```python
from build123d import *

# Parameters (mm, degrees)
EXTRUDE_1_DEPTH          = 16.25
EXTRUDE_1_DEPTH_BACK     = 16.25
SKETCH_2_R               = 1.5
CUT_EXTRUDE_1_DEPTH      = 39.484574832
CUT_EXTRUDE_1_DEPTH_BACK = 39.484574832
SKETCH_3_R               = 1
FILLET_1_R               = 2
CHAMFER_1_SIZE           = 1
SKETCH_4_W               = 8.5
SKETCH_4_H               = 4
CUT_EXTRUDE_2_DEPTH      = 39.484574832


with BuildPart() as part:
    # Sketch 2 → Extrude 1 (new, two sides: drawn at the far end of the back side and taken through both)
    with BuildSketch(Plane(origin=(0, 0, 0), x_dir=(1, 0, 0), z_dir=(0, 1, 0)).offset(-EXTRUDE_1_DEPTH_BACK)):
        with BuildLine():
            Line((-31, 16), (-31, -16))
            Line((-31, -16), (0, -16))
            ThreePointArc((0, -16), (6.583005244, -14.583005244), (12, -10.583005244))
            Line((12, -10.583005244), (12, 10.583005244))
            ThreePointArc((12, 10.583005244), (6.583005244, 14.583005244), (0, 16))
            Line((0, 16), (-31, 16))
        make_face()
        with Locations(Location((0, 0, 0), (0, 0, 270))):
            Circle(SKETCH_2_R, mode=Mode.SUBTRACT)
    extrude(amount=EXTRUDE_1_DEPTH + EXTRUDE_1_DEPTH_BACK)

    # Sketch 3 → Cut-Extrude 1 (cut, two sides: drawn at the far end of the back side and taken through both)
    with BuildSketch(Plane(origin=(0, 0, 0), x_dir=(1, 0, 0), z_dir=(0, 1, 0)).offset(-CUT_EXTRUDE_1_DEPTH_BACK)):
        with Locations(Location((-28, 13.5, 0), (0, 0, 270))):
            Circle(SKETCH_3_R)
        with Locations(Location((-1, 13.5, 0), (0, 0, 270))):
            Circle(SKETCH_3_R)
        with Locations(Location((-1, -13.5, 0), (0, 0, 270))):
            Circle(SKETCH_3_R)
        with Locations(Location((-28, -13.5, 0), (0, 0, 270))):
            Circle(SKETCH_3_R)
    extrude(amount=CUT_EXTRUDE_1_DEPTH + CUT_EXTRUDE_1_DEPTH_BACK, mode=Mode.SUBTRACT)

    # Fillet 1
    fillet_1_edges = [part.edges().sort_by_distance(p)[0] for p in [
        (12, 0, -10.583005244),
        (12, 0, 10.583005244),
        (-31, 0, 16),
        (-31, 0, -16),
    ]]
    fillet(fillet_1_edges, radius=FILLET_1_R)

    # Chamfer 1
    chamfer_1_edges = [part.edges().sort_by_distance(p)[0] for p in [
        (6.198278861, 16.25, 14.750638602),
        (6.198278861, -16.25, 14.750638602),
        (12, 16.25, 0),
        (12, -16.25, 0),
        (6.198278861, 16.25, -14.750638602),
        (-14.5, 16.25, -16),
        (-31, 16.25, 0),
        (-14.5, 16.25, 16),
        (-30.414213562, 16.25, 15.414213562),
        (-30.414213562, 16.25, -15.414213562),
        (11.8516402, 16.25, 10.553887917),
        (11.8516402, 16.25, -10.553887917),
        (6.198278861, -16.25, -14.750638602),
        (-14.5, -16.25, 16),
        (-31, -16.25, 0),
        (-14.5, -16.25, -16),
        (-30.414213562, -16.25, 15.414213562),
        (-30.414213562, -16.25, -15.414213562),
        (11.8516402, -16.25, 10.553887917),
        (11.8516402, -16.25, -10.553887917),
    ]]
    chamfer(chamfer_1_edges, length=CHAMFER_1_SIZE)

    # Sketch 4 → Cut-Extrude 2 (cut, through all)
    with BuildSketch(Plane.XY):
        with Locations((-7.75, -13.15)):
            Rectangle(SKETCH_4_W, SKETCH_4_H)
    extrude(amount=-CUT_EXTRUDE_2_DEPTH, mode=Mode.SUBTRACT)


solid = part.part
```
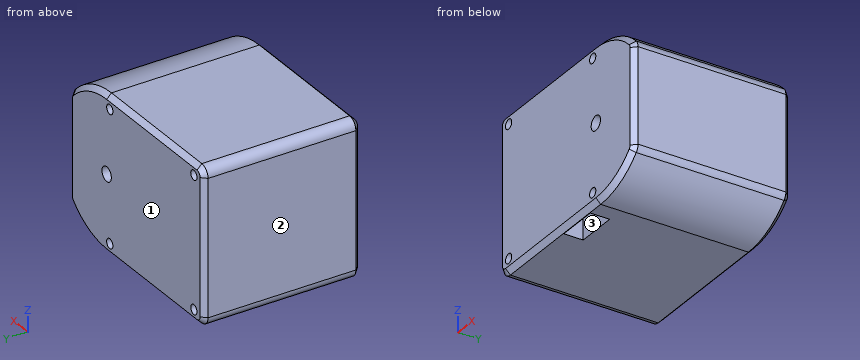
Here's how the part is built. I have some questions about the finished solid (model axes, mm). Face numbers are marked on the shaded views. Give positions to 0.01 mm unless a question says otherwise; leave off trailing zeros. Order: outer loops, then holes, each group sorted by start corner. A loop starts at its lowest first (then second) coordinate and runs counter-clockwise, first axis right, second up. Notation, with made-up numbers: M 45,81.25 L 68,81.25 A26 ccw 68,98.25 Z; hole C 31,-12.5 d9. An arc over 180 degrees is marked long. Use a Markdown table: item, result. Add a question column.
1. Suppose I cut it at C-C (z = -8). List the corners of the cut face in (x, y) for me.
2. If we mould it in two halves opening along Y, with no side actions, what happens to the marked faces 1, 2 and 3? For each: +Y half, -Y half, draft (parallel to the pull), parting line (faces both ways), or undercut.
3. For pin 1 Ø1.2 at (x, y) = (-7, -14) entering from -Z; pin 2 Ø3 at (x, z) = (-1, 13.5) entering from -Y, each with a flat end and sliding along its axis, tell me the tip position at first contact or that it passes through.
4. Suppose I cut it at B-B (y = 8). List the corners of the cut face in (x, z) for me, and give its area (3 significant figures).
5. Suppose I cut it at A-A (x = -28). List the corners of the cut face in (y, z) for me, and give its area (3 significant figures).
6. I need wall thicknesses on probe 1 along Z at (x, y) = (-28, -6); probe 2 along X at (y, z) = (9.5, -13.5); probe 3 along Y at (x, z) = (-8, -8.5). Which ranges of each line are inside material? Lowest first, please. Write a range as from..to.
7. Suppose I cut it at D-D (y = -14). List the corners of the cut face in (x, z) for me.
Results list:
| question | item | result |
|---|---|---|
| 1 | outline | M -31,-15.25 L -30,-16.25 L 11,-16.25 L 12,-15.25 L 12,15.25 L 11,16.25 L -30,16.25 L -31,15.25 Z; hole M -12,-15.15 L -3.5,-15.15 L -3.5,-11.15 L -12,-11.15 Z |
| 2 | face 1 | +Y half |
| 2 | face 2 | draft |
| 2 | face 3 | undercut |
| 3 | pin 1 | stops at z = 0 |
| 3 | pin 2 | stops at y = -16.25 |
| 4 | outline | M -31,-14 A2 ccw -29,-16 L 0,-16 A16 ccw 11.43,-11.2 A2 ccw 12,-9.8 L 12,9.8 A2 ccw 11.43,11.2 A16 ccw 0,16 L -29,16 A2 ccw -31,14 Z; hole C -28,-13.5 d2; hole C -28,13.5 d2; hole C -1,-13.5 d2; hole C -1,13.5 d2; hole C 0,0 d3 |
| 4 | area | 1,310 mm² |
| 5 | outline | M -16.25,-15 L -15.25,-16 L 15.25,-16 L 16.25,-15 L 16.25,-14.5 L -16.25,-14.5 Z; M -16.25,-12.5 L 16.25,-12.5 L 16.25,12.5 L -16.25,12.5 Z; M -16.25,14.5 L 16.25,14.5 L 16.25,15 L 15.25,16 L -15.25,16 L -16.25,15 Z |
| 5 | area | 908 mm² |
| 6 | probe 1 | z = -16..-14.5, -12.5..12.5, 14.5..16 |
| 6 | probe 2 | x = -31..-29, -27..-2, 0..8.59 |
| 6 | probe 3 | y = -16.25..-15.15, -11.15..16.25 |
| 7 | outline | M -31,-14 A2 ccw -29,-16 L -12,-16 L -12,0 L -3.5,0 L -3.5,-16 L 0,-16 A16 ccw 11.43,-11.2 A2 ccw 12,-9.8 L 12,9.8 A2 ccw 11.43,11.2 A16 ccw 0,16 L -29,16 A2 ccw -31,14 Z; hole C -28,-13.5 d2; hole C -28,13.5 d2; hole C -1,-13.5 d2; hole C -1,13.5 d2; hole C 0,0 d3 |
